Model file for the job. Use its own axes, mm. A direction names the side the tool comes from. Round coordinates to 2 decimals unless told otherwise and drop trailing zeros. Loops run counter-clockwise (first coordinate to the right, second up) from the corner with the lowest first, then second, coordinate; pieces in that order, holes last. Notation, with made-up numbers: (79.5, -12) - (101.5, -12) arc R27 cw to (101.5, 11) - close; hole circle Ø11 at (73.25, 3). An arc over 180 degrees is marked (long way). Answer as a JSON object with one key per item and string values.
from build123d import *

# Parameters (mm, degrees)
SKETCH1_W           = 38.1
SKETCH1_H           = 50.8
BOSS_EXTRUDE1_DEPTH = 5.08
SKETCH2_R           = 6.35
SKETCH2_R_2         = 1.8288
CUT_EXTRUDE1_DEPTH  = 5.08
SKETCH3_W           = 5.08
SKETCH3_H           = 5.08
BOSS_EXTRUDE2_DEPTH = 5.08
SKETCH4_W           = 38.1
SKETCH4_H           = 5.08
CUT_EXTRUDE2_DEPTH  = 11.43


with BuildPart() as part:
    # Sketch1 → Boss-Extrude1 (new body)
    with BuildSketch(Plane.XY):
        with Locations((2.494642857, -9.638392857)):
            Rectangle(SKETCH1_W, SKETCH1_H)
    extrude(amount=BOSS_EXTRUDE1_DEPTH)

    # Sketch2 → Cut-Extrude1 (cut)
    with BuildSketch(Plane.XY.offset(5.08)):
        with Locations((2.494642857, -9.638392857)):
            Circle(SKETCH2_R)
        with Locations((12.273642857, -9.638392857)):
            Circle(SKETCH2_R_2)
        with Locations((9.40944007, -16.55319007)):
            Circle(SKETCH2_R_2)
        with Locations((2.494642857, -19.417392857)):
            Circle(SKETCH2_R_2)
        with Locations((-4.420154356, -16.55319007)):
            Circle(SKETCH2_R_2)
        with Locations((-7.284357143, -9.638392857)):
            Circle(SKETCH2_R_2)
        with Locations((-4.420154356, -2.723595644)):
            Circle(SKETCH2_R_2)
        with Locations((2.494642857, 0.140607143)):
            Circle(SKETCH2_R_2)
        with Locations((9.40944007, -2.723595644)):
            Circle(SKETCH2_R_2)
    extrude(amount=-CUT_EXTRUDE1_DEPTH, mode=Mode.SUBTRACT)

    # Sketch3 → Boss-Extrude2 (add)
    with BuildSketch(Plane.XY.offset(5.08)):
        with Locations((-14.015357143, 18.301607143)):
            Rectangle(SKETCH3_W, SKETCH3_H)
        with Locations((8.844642857, 18.301607143)):
            Rectangle(SKETCH3_W, SKETCH3_H)
        with Locations((19.004642857, 18.301607143)):
            Rectangle(SKETCH3_W, SKETCH3_H)
        with Locations((-3.855357143, 18.301607143)):
            Rectangle(SKETCH3_W, SKETCH3_H)
        with Locations((-3.855357143, -37.578392857)):
            Rectangle(SKETCH3_W, SKETCH3_H)
        with Locations((-14.015357143, -37.578392857)):
            Rectangle(SKETCH3_W, SKETCH3_H)
        with Locations((19.004642857, -37.578392857)):
            Rectangle(SKETCH3_W, SKETCH3_H)
        with Locations((8.844642857, -37.578392857)):
            Rectangle(SKETCH3_W, SKETCH3_H)
    extrude(amount=-BOSS_EXTRUDE2_DEPTH)

    # Sketch4 → Cut-Extrude2 (cut)
    with BuildSketch(Plane.XZ.offset(40.118392857)):
        with Locations((2.494642857, 2.54)):
            Rectangle(SKETCH4_W, SKETCH4_H)
    extrude(amount=-CUT_EXTRUDE2_DEPTH, mode=Mode.SUBTRACT)


solid = part.part
1) Slice it at A-A on x = -8.5. List the corners of the cut face in (y, z), then the cut area to 3 significant figures.
Values follow:
{"outline": "(-28.69, 0) - (-11, 0) - (-11, 5.08) - (-28.69, 5.08) - close; (-8.27, 0) - (15.76, 0) - (15.76, 5.08) - (-8.27, 5.08) - close", "area": "212 mm²"}
2) Probe probe 1 along Y at (x, z) = (-6, 4.1); probe 2 along X at (y, z) = (-16.5, 1.8); probe 3 along X at (y, z) = (-18, 2.2). List the from-to ranges inside material, lowest first.
Values follow:
{"probe 1": "-28.69 to -17.47, -15.63 to -10.94, -8.34 to -3.64, -1.8 to 20.84", "probe 2": "-16.56 to -6.25, -2.59 to 7.58, 11.24 to 21.54", "probe 3": "-16.56 to -5.54, -3.3 to 1.34, 3.65 to 8.29, 10.53 to 21.54"}
3) Two-plate mould, pull along X, no slides. Class faces 3 (the cylindrical face through (-2.73, -3.42, 2.58)), 4 (the flat face through (19, 20.842, 3)), 5 (the flat face through (21.545, -4, 3)): pulls with the +X half, pulls with the -X half, needs draft (parallel to the pull), parting line crosses it, or undercut.
Values follow:
{"face 3": "undercut", "face 4": "needs draft", "face 5": "pulls with the +X half"}
4) Tool access for faces 1 (the flat face through (11.385, 18, 3)), 2 (the cylindrical face through (-4.66, -14.74, 2.58)): list every direction of +Z, -Z, +X, -X, +Y, -Y with a clear straight run to the whole face (end or side of a thin tool).
Values follow:
{"face 1": "+Z, -Z, +Y", "face 2": "+Z, -Z"}
5) Slice it at B-B on y = -12. List the corners of the cut face in (x, z).
Values follow:
{"outline": "(-16.56, 0) - (-3.4, 0) - (-3.4, 5.08) - (-16.56, 5.08) - close; (8.39, 0) - (21.54, 0) - (21.54, 5.08) - (8.39, 5.08) - close"}
6) Slice it at C-C on z = 1.8. Count the separate pieces of the cut face and the enclosed holes in it, then the cut area to 3 significant figures.
Values follow:
{"separate pieces": "1", "enclosed holes": "9", "area": "1,590 mm²"}
7) Slice it at D-D on x = 2. List the corners of the cut face in (y, z).
Values follow:
{"outline": "(-28.69, 0) - (-21.18, 0) - (-21.18, 5.08) - (-28.69, 5.08) - close; (-17.66, 0) - (-15.97, 0) - (-15.97, 5.08) - (-17.66, 5.08) - close; (-3.31, 0) - (-1.62, 0) - (-1.62, 5.08) - (-3.31, 5.08) - close; (1.9, 0) - (15.76, 0) - (15.76, 5.08) - (1.9, 5.08) - close"}
